```python
from build123d import *

# Parameters (mm, degrees)
BASE_FLANGE1_DEPTH          = 44.45
LONG_SLOT_DEPTH             = 170.46496681
SHORT_SLOT_DEPTH            = 170.46496681
LPATTERN1_COUNT             = 2
LPATTERN1_PITCH             = 57.15
LPATTERN2_COUNT             = 2
LPATTERN2_PITCH             = 63.5
LPATTERN2_COUNT_DIR2        = 2
LPATTERN2_PITCH_DIR2        = 50.8
F_1_4_0_25_DIAMETER_HOLE1_D = 6.35
FILLET1_R                   = 12.7


# Sheet-metal steps are written as plain solids
with BuildPart() as part:
    # Sketch1 → Base-Flange1 (new, symmetric)
    with BuildSketch(Plane.XY):
        with BuildLine():
            Line((139.7, 0), (13.41628, 0))
            ThreePointArc((13.41628, 0), (3.929537434, 3.929537434), (0, 13.41628))
            Line((0, 13.41628), (0, 88.9))
            Line((0, 88.9), (3.89128, 88.9))
            Line((3.89128, 88.9), (3.89128, 13.41628))
            ThreePointArc((3.89128, 13.41628), (6.681087909, 6.681087909), (13.41628, 3.89128))
            Line((13.41628, 3.89128), (139.7, 3.89128))
            Line((139.7, 3.89128), (139.7, 0))
        make_face()
    extrude(amount=BASE_FLANGE1_DEPTH, both=True)

    # Sketch4 → LONG-SLOT (cut, through all)
    with BuildSketch(Plane(origin=(0, 3.89128, 0), x_dir=(1, 0, 0), z_dir=(0, 1, 0))):
        with BuildLine():
            Line((25.781, 5.1562), (128.1938, 5.1562))
            ThreePointArc((128.1938, 5.1562), (133.35, 0), (128.1938, -5.1562))
            Line((128.1938, -5.1562), (25.781, -5.1562))
            ThreePointArc((25.781, -5.1562), (20.6248, 0), (25.781, 5.1562))
        make_face()
    extrude(amount=-LONG_SLOT_DEPTH, mode=Mode.SUBTRACT)

    # Sketch5 → SHORT-SLOT (cut, through all)
    with BuildSketch(Plane(origin=(0, 3.89128, 0), x_dir=(1, 0, 0), z_dir=(0, 1, 0))):
        with BuildLine():
            Line((51.9938, -23.0378), (128.1938, -23.0378))
            ThreePointArc((128.1938, -23.0378), (133.35, -28.194), (128.1938, -33.3502))
            Line((128.1938, -33.3502), (51.9938, -33.3502))
            ThreePointArc((51.9938, -33.3502), (46.8376, -28.194), (51.9938, -23.0378))
        make_face()
    short_slot = extrude(amount=-SHORT_SLOT_DEPTH, mode=Mode.SUBTRACT)

    # LPattern1: SHORT-SLOT ×2
    with Locations(*[(0, 0, -i * LPATTERN1_PITCH) for i in range(1, LPATTERN1_COUNT)]):
        add(short_slot, mode=Mode.SUBTRACT)

    # Sketch6 → CSK for 1/4 Flat Head Machine Screw1 (revolve, cut)
    with BuildSketch(Plane(origin=(3.89128, 76.2, 31.75), x_dir=(0, 0, -1), z_dir=(0, 1, 0))):
        Polygon((0, 0), (0, 3.89128), (3.57124, 3.89128), (3.57124, 3.298865467), (6.4389, 0), align=None)
    csk_for_1_4_flat_head_machine_screw1 = revolve(axis=Axis((10.24128, 76.2, 31.75), (-1, 0, 0)), mode=Mode.SUBTRACT)

    # LPattern2: CSK for 1_4 Flat Head Machine Screw1 2 × 2
    with Locations(*[(0, -j * LPATTERN2_PITCH_DIR2, -i * LPATTERN2_PITCH) for i in range(LPATTERN2_COUNT) for j in range(LPATTERN2_COUNT_DIR2) if (i, j) != (0, 0)]):
        add(csk_for_1_4_flat_head_machine_screw1, mode=Mode.SUBTRACT)

    # 1/4 (0.25) Diameter Hole1 (through all)
    with Locations(Plane(origin=(3.89128, 0, 0), x_dir=(0, 0, -1), z_dir=(1, 0, 0))):
        with Locations((-28.575, 60.325), (14.2748, 73.025)):
            Hole(F_1_4_0_25_DIAMETER_HOLE1_D / 2)

    # Fillet1
    fillet1_edges = [part.edges().sort_by_distance(p)[0] for p in [
        (139.7, 1.94564, 44.45),
        (139.7, 1.94564, -44.45),
    ]]
    fillet(fillet1_edges, radius=FILLET1_R)


solid = part.part
```
Work out the finished part from the listing and answer in its coordinate system (mm). A direction names the side the tool comes from. Coordinates: 2 decimals unless noted, no trailing zeros. Loops run counter-clockwise (first coordinate to the right, second up) from the corner with the lowest first, then second, coordinate; pieces in that order, holes last. Notation, with made-up numbers: (14, -18.75) -> (40, -18.75) arc R18 cw to (40, -13.75) -> close; hole circle Ø5 at (29, 54). An arc over 180 degrees is marked (long way). Answer as CSV lines item,"result".
Q1. A tool of negligible diameter and unlimited length cuts with its end or side. For faces 5 (the face through (4.03, 3.83, 0.62)), 6 (the face through (133.35, 1.97, -29.07)), from which of +Z, -Z, +X, -X, +Y, -Y can it reach the whole face along a straight path? Write none if from no direction.
Findings:
face 5,"+Z, -Z, -X, -Y"
face 6,"+Y, -Y"
Q2. The part is cut by section B-B on y = 25.4. Write down the section's boundary in (x, z).
Findings:
outline,"(0, -44.45) -> (3.89, -44.45) -> (3.89, -38.19) -> (0.59, -35.32) -> (0, -35.32) -> close; (0, -28.18) -> (0.59, -28.18) -> (3.89, -25.31) -> (3.89, 25.31) -> (0.59, 28.18) -> (0, 28.18) -> close; (0, 35.32) -> (0.59, 35.32) -> (3.89, 38.19) -> (3.89, 44.45) -> (0, 44.45) -> close"
Q3. The part is cut by section A-A on z = 0. Write down the section's boundary in (x, y) (3 decimals).
Findings:
outline,"(0, 13.416) arc R13.416 ccw to (13.416, 0) -> (20.625, 0) -> (20.625, 3.891) -> (13.416, 3.891) arc R9.525 cw to (3.891, 13.416) -> (3.891, 88.9) -> (0, 88.9) -> close; (133.35, 0) -> (139.7, 0) -> (139.7, 3.891) -> (133.35, 3.891) -> close"
Q4. The part is cut by section C-C on x = 63. Write down the section's boundary in (y, z), and give its area (3 significant figures).
Findings:
outline,"(0, -44.45) -> (3.89, -44.45) -> (3.89, -34.11) -> (0, -34.11) -> close; (0, -23.8) -> (3.89, -23.8) -> (3.89, -5.16) -> (0, -5.16) -> close; (0, 5.16) -> (3.89, 5.16) -> (3.89, 23.04) -> (0, 23.04) -> close; (0, 33.35) -> (3.89, 33.35) -> (3.89, 44.45) -> (0, 44.45) -> close"
area,"226 mm²"
Q5. The part is cut by section D-D on z = -19. Write down the section's boundary in (x, y) (3 decimals), and give its area (3 significant figures).
Findings:
outline,"(0, 13.416) arc R13.416 ccw to (13.416, 0) -> (139.7, 0) -> (139.7, 3.891) -> (13.416, 3.891) arc R9.525 cw to (3.891, 13.416) -> (3.891, 88.9) -> (0, 88.9) -> close"
area,"855 mm²"
Q6. For a pull along X with two mould halves and no side action, classify faces 1 (the face through (46.84, 1.97, -28.84)), 2 (the face through (91, 2, -23.8)), 3 (the face through (0.799, 29.061, -30.937)), 4 (the face through (76, 3.891, 11)) as +X half, -X half, draft (parallel to the pull), parting line (faces both ways), or undercut.
Findings:
face 1,"undercut"
face 2,"undercut"
face 3,"+X half"
face 4,"draft"
Q7. Find the intervals of material crossed by probe 1 along X at (y, z) = (41, 19); probe 2 along Y at (x, z) = (10, -23.5), in increasing order.
Findings:
probe 1,"x = 0 to 3.89"
probe 2,"y = 0.44 to 4.53"
Q8. Each of these flat-tipped pins is pushed along its axis until it touches: pin 1 (1 mm diameter, centred on y = 64, z = 3.5, fed in from +X); pin 2 (8 mm diameter, centred on x = 20, z = -6, fed in from +Y); pin 3 (4 mm diameter, centred on x = 93, z = 5.5, fed in from -Y); pin 4 (4.5 mm diameter, centred on y = 25.4, z = 31.75, fed in from +X). Where does it stop, or does it pass through?
Findings:
pin 1,"stops at x = 3.89"
pin 2,"stops at y = 3.89"
pin 3,"stops at y = 0"
pin 4,"passes through"
